Source: CAD feature listing. Evaluate the final solid. Frame: model axes, mm. Face numbers are marked on the shaded views. A direction names the side the tool comes from. Round coordinates to 2 decimals unless told otherwise and drop trailing zeros. Loops run counter-clockwise (first coordinate to the right, second up) from the corner with the lowest first, then second, coordinate; pieces in that order, holes last.
(1) Set-up query: the marked faces 1, 2 and 3. Return all of +Z, -Z, +X, -X, +Y, -Y with unobstructed straight access to the full face (end or side cutting, diameter ignored); none if empty.
(2) First-contact query: pin 1 Ø4 at (x, z) = (-58, 35.5) entering from +Y; pin 2 Ø3 at (x, y) = (-19.5, -14) entering from -Z; pin 3 Ø4 at (x, z) = (22.86, 0) entering from +Y. Flat tips, straight axial feed; report the tip coordinate or a pass-through.
(3) Section C-C, the plane x = -53. Return the cut outline in (y, z), plus the area to 3 significant figures.
(4) Material intervals for probe 1 along X at (y, z) = (1, 0); probe 2 along Z at (x, y) = (22.86, 1.3); probe 3 along Z at (x, y) = (-32.5, -53), sorted ascending.
(5) Section A-A, the plane z = 0. Count the separate pieces of the cut face and the enclosed holes in it, plus the area to 3 significant figures.
(6) Section B-B, the plane z = -41.5. Return the cut outline in (x, y), plus the area to 3 significant figures.
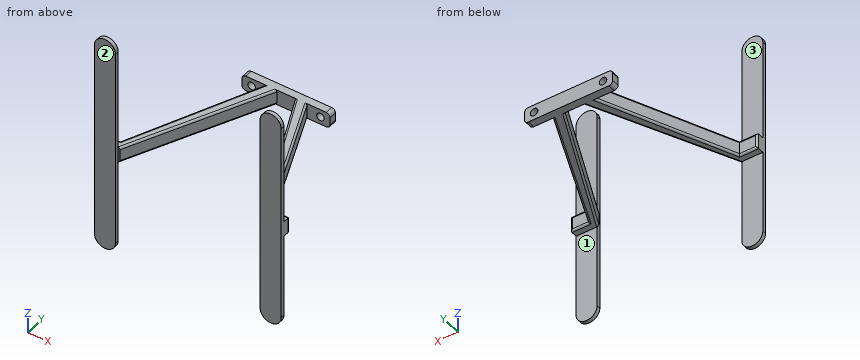
```python
from build123d import *

# Parameters (mm, degrees)
SKETCH1_R           = 2.5
BOSS_EXTRUDE1_DEPTH = 5.08
BOSS_EXTRUDE2_DEPTH = 10.16
FILLET2_R           = 1.27
FILLET3_R           = 1.27
BOSS_EXTRUDE3_DEPTH = 2.54


with BuildPart() as part:
    # Sketch1 → Boss-Extrude1 (new body)
    with BuildSketch(Plane(origin=(0, 0, 0), x_dir=(1, 0, 0), z_dir=(0, 1, 0))):
        with BuildLine():
            Line((26.705849829, 5.08), (-26.705849829, 5.08))
            ThreePointArc((-26.705849829, 5.08), (-28.501901053, 4.336051224), (-29.245849829, 2.54))
            Line((-29.245849829, 2.54), (-29.245849829, -2.54))
            ThreePointArc((-29.245849829, -2.54), (-28.501901053, -4.336051224), (-26.705849829, -5.08))
            Line((-26.705849829, -5.08), (26.705849829, -5.08))
            ThreePointArc((26.705849829, -5.08), (28.501901053, -4.336051224), (29.245849829, -2.54))
            Line((29.245849829, -2.54), (29.245849829, 2.54))
            ThreePointArc((29.245849829, 2.54), (28.501901053, 4.336051224), (26.705849829, 5.08))
        make_face()
        with Locations(Location((-22.86, 0, 0), (0, 0, 270))):
            Circle(SKETCH1_R, mode=Mode.SUBTRACT)
        with Locations(Location((22.86, 0, 0), (0, 0, 90))):
            Circle(SKETCH1_R, mode=Mode.SUBTRACT)
    extrude(amount=BOSS_EXTRUDE1_DEPTH)

    # Sketch2 → Boss-Extrude2 (add)
    with BuildSketch(Plane.XY.offset(5.08)):
        Polygon((-14.007084232, 0), (-50.125026448, -84.328), (-61.947051412, -84.328), (-61.947051412, -89.408), (-50.8, -89.408), (-46.892843325, -89.408), (-6.12233164, 0), align=None)
        Polygon((50.8, -89.408), (61.947051412, -89.408), (61.947051412, -84.328), (50.125026448, -84.328), (14.007084232, 0), (6.12233164, 0), (46.892843325, -89.408), align=None)
    extrude(amount=-BOSS_EXTRUDE2_DEPTH)

    # Fillet2
    fillet2_edges = [part.edges().sort_by_distance(p)[0] for p in [
        (-56.03603893, -84.328, -5.08),
        (-61.947051412, -84.328, 0),
        (-56.03603893, -84.328, 5.08),
        (56.03603893, -84.328, -5.08),
        (61.947051412, -84.328, 0),
        (56.03603893, -84.328, 5.08),
    ]]
    fillet(fillet2_edges, radius=FILLET2_R)

    # Fillet3
    fillet3_edges = [part.edges().sort_by_distance(p)[0] for p in [
        (32.338027797, -42.799, 5.08),
        (26.507587483, -44.704, 5.08),
        (26.507587483, -44.704, -5.08),
        (32.338027797, -42.799, -5.08),
        (-26.507587483, -44.704, 5.08),
        (-26.507587483, -44.704, -5.08),
        (-32.338027797, -42.799, -5.08),
        (-32.338027797, -42.799, 5.08),
    ]]
    fillet(fillet3_edges, radius=FILLET3_R)

    # Sketch3 → Boss-Extrude3 (add)
    with BuildSketch(Plane.XZ.offset(89.408)):
        with BuildLine():
            Line((47.98747777, 72.005934115), (47.98747777, -60.440977769))
            ThreePointArc((47.98747777, -60.440977769), (54.967264591, -67.420764589), (61.947051412, -60.440977769))
            Line((61.947051412, -60.440977769), (61.947051412, 72.005934115))
            ThreePointArc((61.947051412, 72.005934115), (54.967264591, 78.985720936), (47.98747777, 72.005934115))
        make_face()
        with BuildLine():
            Line((-61.947051412, 72.005934115), (-61.947051412, -60.440977769))
            ThreePointArc((-61.947051412, -60.440977769), (-54.967264591, -67.420764589), (-47.98747777, -60.440977769))
            Line((-47.98747777, -60.440977769), (-47.98747777, 72.005934115))
            ThreePointArc((-47.98747777, 72.005934115), (-54.967264591, 78.985720936), (-61.947051412, 72.005934115))
        make_face()
    extrude(amount=BOSS_EXTRUDE3_DEPTH)


solid = part.part
```
Output values:
1. face 1: -Z, +X, -X, +Y
1. face 2: +Z, -Z, +X, -X, -Y
1. face 3: +Z, +X, -X, +Y
2. pin 1: stops at y = -89.41
2. pin 2: stops at z = -5.08
2. pin 3: stops at y = -16
3. outline: (-91.95, -67.14) - (-89.41, -67.14) - (-89.41, -5.08) - (-85.6, -5.08) arc R1.27 ccw to (-84.33, -3.81) - (-84.33, 3.81) arc R1.27 ccw to (-85.6, 5.08) - (-89.41, 5.08) - (-89.41, 78.7) - (-91.95, 78.7) - close
3. area: 421 mm2
4. probe 1: x = -29.25 to -25.36, -20.36 to 20.36, 25.36 to 29.25
4. probe 2: z = -5.08 to -2.5, 2.5 to 5.08
4. probe 3: z = -5.08 to 5.08
5. separate pieces: 3
5. enclosed holes: 0
5. area: 1,610 mm2
6. outline: (-61.95, -91.95) - (-47.99, -91.95) - (-47.99, -89.41) - (-61.95, -89.41) - close; (47.99, -91.95) - (61.95, -91.95) - (61.95, -89.41) - (47.99, -89.41) - close
6. area: 70.9 mm2
